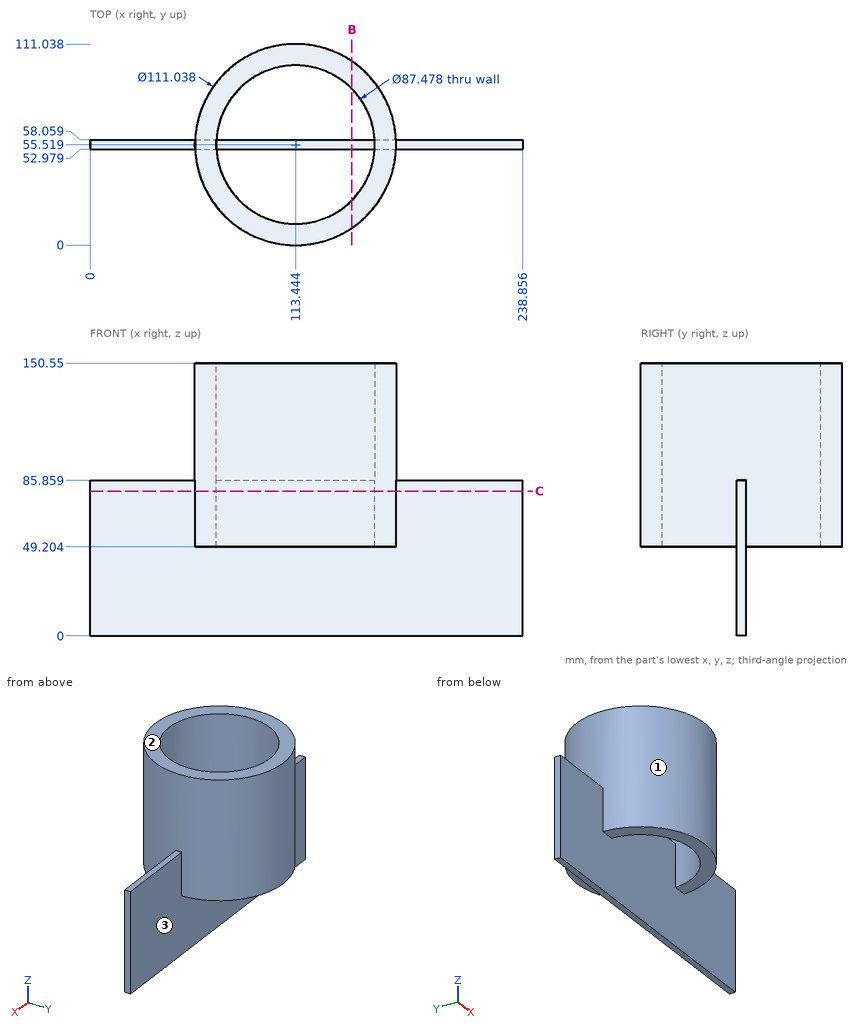
Design review of the part shown in the three views and the two pictorial views. Dimensions are in mm from the part's minimum x, y and z. Round coordinates to 2 decimals unless told otherwise and drop trailing zeros. Write each loop counter-clockwise with the first axis right and the second up, starting at its lowest first coordinate (ties: lowest second). Pieces come first, ordered by that corner, then holes.
Item 1: The part is to be moulded in two halves that separate along X. For the marked faces 1, 2 and 3, say which applies: +X half, -X half, draft (parallel to the pull), parting line (faces both ways), or undercut.
Item 2: We need section B-B on x = 144.5. State how many separate pieces and enclosed holes the cut face has, and give its area (3 significant figures).
Item 3: For probe 1 along X at (y, z) = (29, 80) (1 decimal); probe 2 along Y at (x, z) = (198, 67); probe 3 along X at (y, z) = (94.5, 110.5) (1 decimal), list the stretches that pass through material, from the lowest coordinate up.
Item 4: We need section C-C on z = 80. Write out the cut boundary in (x, y) (1 decimal), and give its area (3 significant figures).
Item 5: Clearance check with flat-ended pins moving along their axes: pin 1 Ø5 at (x, z) = (188.5, 79) entering from +Y; pin 2 Ø2.5 at (x, y) = (114.5, 54.5) entering from +Z; pin 3 Ø12 at (x, z) = (188, 49.5) entering from -Y. State where each tip first meets the part, or that it passes through.
Returned:
1. face 1: parting line
1. face 2: draft
1. face 3: undercut
2. separate pieces: 3
2. enclosed holes: 0
2. area: 3,520 mm2
3. probe 1: x = 64.7 to 78.7, 148.2 to 162.2
3. probe 2: y = 52.98 to 58.06
3. probe 3: x = 73.9 to 93.6, 133.3 to 153
4. outline: (0, 53) - (58, 53) arc R55.5 ccw to (168.9, 53) - (238.9, 53) - (238.9, 58.1) - (168.9, 58.1) arc R55.5 ccw to (58, 58.1) - (0, 58.1) - close; hole (69.8, 53) arc R43.7 ccw to (157.1, 53) - close; hole (69.8, 58.1) - (157.1, 58.1) arc R43.7 ccw to start
4. area: 4,770 mm2
5. pin 1: stops at y = 58.06
5. pin 2: stops at z = 85.86
5. pin 3: stops at y = 52.98
